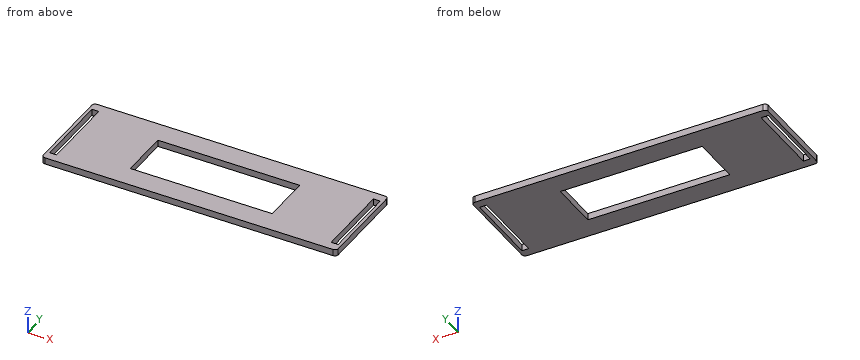
Autodesk Inventor part; units mm, degrees
ref_plane "YZ Plane" through (0, 0, 0) normal (1, 0, 0) x (0, 1, 0)
ref_plane "XZ Plane" through (0, 0, 0) normal (0, 1, 0) x (-1, 0, 0)
ref_plane "XY Plane" through (0, 0, 0) normal (0, 0, 1) x (1, 0, 0)
sketch "Sketch1" plane through (0, 0, 0) normal (0, 0, 1) x (1, 0, 0)
  line L0 (-134, -42.5) -> (134, -42.5)
  line L1 (134, -42.5) -> (134, 42.5)
  line L2 (134, 42.5) -> (-134, 42.5)
  line L3 (-134, 42.5) -> (-134, -42.5)
  line L4 (-134, -42.5) -> (134, 42.5) construction
  line L5 (134, -42.5) -> (-134, 42.5) construction
  point P0 (0, 0)
  dimension "d0" = 85
  dimension "d1" = 268
extrude "Extrusion1" add sketch "Sketch1" along normal blind 6
sketch "Sketch2" plane through (0, 0, 6) normal (0, 0, 1) x (1, 0, 0)
  line L0 (-134, -42.5) -> (134, -42.5)
  line L1 (134, -42.5) -> (134, 42.5)
  line L2 (-131.125, -34.5) -> (-124.875, -34.5)
  line L3 (-124.875, -34.5) -> (-124.875, 34.5)
  line L4 (-124.875, 34.5) -> (-131.125, 34.5)
  line L5 (-131.125, 34.5) -> (-131.125, -34.5)
  line L6 (-131.125, -34.5) -> (-124.875, 34.5) construction
  line L7 (-124.875, -34.5) -> (-131.125, 34.5) construction
  line L8 (124.875, -34.5) -> (131.125, -34.5)
  line L9 (131.125, -34.5) -> (131.125, 34.5)
  line L10 (131.125, 34.5) -> (124.875, 34.5)
  line L11 (124.875, 34.5) -> (124.875, -34.5)
  line L12 (124.875, -34.5) -> (131.125, 34.5) construction
  line L13 (131.125, -34.5) -> (124.875, 34.5) construction
  line L14 (134, 42.5) -> (-134, 42.5)
  line L15 (-134, 42.5) -> (-134, -42.5)
  point P0 (0, 0)
  point P1 (-128, 0)
  point P2 (128, 0)
  dimension "d5" = 2.875
  dimension "d6" = 6.25
  dimension "d8" = 8
  dimension "d34" = 2.875
  dimension "d35" = 8
extrude "Extrusion2" cut sketch "Sketch2" against normal through all contours L5 L4 L3 L2 | L11 L10 L9 L8
fillet "Fillet1" radius 3 4 edges at (134, -42.5, 3) (134, 42.5, 3) (-134, -42.5, 3) (-134, 42.5, 3)
sketch "Sketch4" plane through (0, 0, 6) normal (0, 0, 1) x (1, 0, 0)
  line L0 (64.5, -22.5) -> (-64.5, -22.5)
  line L1 (-64.5, -22.5) -> (-64.5, 22.5)
  line L2 (-64.5, 22.5) -> (64.5, 22.5)
  line L3 (64.5, 22.5) -> (64.5, -22.5)
  line L4 (64.5, -22.5) -> (-64.5, 22.5) construction
  line L5 (-64.5, -22.5) -> (64.5, 22.5) construction
  line L6 (131, 42.5) -> (-131, 42.5)
  line L7 (-131, -42.5) -> (131, -42.5)
  line L8 (0, -42.5) -> (0, 0) construction
  dimension "d2" = 6
  dimension "d33" = 20
  dimension "d36" = 129
  dimension "d37" = 20
extrude "Extrusion5" cut sketch "Sketch4" against normal blind 10
equation "\"d34\" = d5"
properties part number "TopFrontPanel"
Check sheet for the modelled part. Datum: model origin and axes. Units: mm. Give positions to 0.01 mm unless a question says otherwise; leave off trailing zeros. Loops run counter-clockwise (first coordinate to the right, second up) from the corner with the lowest first, then second, coordinate; pieces in that order, holes last. Notation, with made-up numbers: M 36.25,-11 L 56.25,-11 A13 ccw 56.25,0 Z; hole C 30.25,-18 d1. An arc over 180 degrees is marked long. Return JSON: item names as keys, results as strings. Group by question number.
1. Cross-section at C-C on y = -28. Record the boundary of the cut face in (x, z) (3 decimals), plus the area to 3 significant figures.
2. Cross-section at A-A on y = -17. Record the boundary of the cut face in (x, z) (3 decimals), plus the area to 3 significant figures.
3. Cross-section at D-D on x = 24. Record the boundary of the cut face in (y, z), plus the area to 3 significant figures.
4. Cross-section at B-B on z = 2.4. Record the boundary of the cut face in (x, y) (3 decimals), plus the area to 3 significant figures.
5. Thickness scan on L1, parallel to X at y = 22, z = 5.2 (3 decimals); L2, parallel to X at y = -26, z = 2.55 (3 decimals); L3, parallel to Y at x = -30, z = 4.85. Record the ranges inside material, lowest first.
Return value:
{
 "1": {"outline": "M -134,0 L -131.125,0 L -131.125,6 L -134,6 Z; M -124.875,0 L 124.875,0 L 124.875,6 L -124.875,6 Z; M 131.125,0 L 134,0 L 134,6 L 131.125,6 Z", "area": "1,530 mm^2"},
 "2": {"outline": "M -134,0 L -131.125,0 L -131.125,6 L -134,6 Z; M -124.875,0 L -64.5,0 L -64.5,6 L -124.875,6 Z; M 64.5,0 L 124.875,0 L 124.875,6 L 64.5,6 Z; M 131.125,0 L 134,0 L 134,6 L 131.125,6 Z", "area": "759 mm^2"},
 "3": {"outline": "M -42.5,0 L -22.5,0 L -22.5,6 L -42.5,6 Z; M 22.5,0 L 42.5,0 L 42.5,6 L 22.5,6 Z", "area": "240 mm^2"},
 "4": {"outline": "M -134,-39.5 A3 ccw -131,-42.5 L 131,-42.5 A3 ccw 134,-39.5 L 134,39.5 A3 ccw 131,42.5 L -131,42.5 A3 ccw -134,39.5 Z; hole M -131.125,-34.5 L -124.875,-34.5 L -124.875,34.5 L -131.125,34.5 Z; hole M -64.5,-22.5 L 64.5,-22.5 L 64.5,22.5 L -64.5,22.5 Z; hole M 124.875,-34.5 L 131.125,-34.5 L 131.125,34.5 L 124.875,34.5 Z", "area": "16,100 mm^2"},
 "5": {"L1": "-134 to -131.125, -124.875 to -64.5, 64.5 to 124.875, 131.125 to 134", "L2": "-134 to -131.125, -124.875 to 124.875, 131.125 to 134", "L3": "-42.5 to -22.5, 22.5 to 42.5"}
}
